Model file for the job. Use its own axes, mm. A direction names the side the tool comes from. Give positions to 0.01 mm unless a question says otherwise; leave off trailing zeros. Write each loop counter-clockwise with the first axis right and the second up, starting at its lowest first coordinate (ties: lowest second). Pieces come first, ordered by that corner, then holes.
```python
from build123d import *

# Parameters (mm, degrees)
SKETCH1_W           = 25.4
SKETCH1_H           = 46.164
BOSS_EXTRUDE1_DEPTH = 6.88
SKETCH2_W           = 13.76
SKETCH2_H           = 15
BOSS_EXTRUDE2_DEPTH = 6.88
SKETCH3_R           = 2.55
CUT_EXTRUDE1_DEPTH  = 7.88
CHAMFER1_SIZE       = 2
FILLET1_R           = 2


with BuildPart() as part:
    # Sketch1 → Boss-Extrude1 (new body)
    with BuildSketch(Plane.XY):
        Rectangle(SKETCH1_W, SKETCH1_H)
    extrude(amount=-BOSS_EXTRUDE1_DEPTH)

    # Sketch2 → Boss-Extrude2 (add)
    with BuildSketch(Plane.XY):
        with Locations((-12.7, 0)):
            Rectangle(SKETCH2_W, SKETCH2_H)
    boss_extrude2 = extrude(amount=-BOSS_EXTRUDE2_DEPTH)

    # Mirror2: Boss-Extrude2 across plane
    add(boss_extrude2.mirror(Plane(origin=(0, 0, 0), x_dir=(0, 0, 1), z_dir=(1, 0, 0))))

    # Sketch3 → Cut-Extrude1 (cut, through all)
    with BuildSketch(Plane.XY):
        Circle(SKETCH3_R)
    extrude(amount=-CUT_EXTRUDE1_DEPTH, mode=Mode.SUBTRACT)

    # Chamfer1
    chamfer1_edges = [part.edges().sort_by_distance(p)[0] for p in [
        (-19.58, -7.5, -3.44),
        (-19.58, 7.5, -3.44),
        (19.58, 7.5, -3.44),
        (19.58, -7.5, -3.44),
        (-12.7, 23.082, -3.44),
        (12.7, 23.082, -3.44),
        (12.7, -23.082, -3.44),
        (-12.7, -23.082, -3.44),
    ]]
    chamfer(chamfer1_edges, length=CHAMFER1_SIZE)

    # Fillet1
    fillet1_edges = [part.edges().sort_by_distance(p)[0] for p in [
        (10.7, 23.082, -3.44),
        (-10.7, 23.082, -3.44),
        (-12.7, 21.082, -3.44),
        (-17.58, 7.5, -3.44),
        (-19.58, -5.5, -3.44),
        (-19.58, 5.5, -3.44),
        (-17.58, -7.5, -3.44),
        (-12.7, -21.082, -3.44),
        (10.7, -23.082, -3.44),
        (-10.7, -23.082, -3.44),
        (12.7, -21.082, -3.44),
        (17.58, -7.5, -3.44),
        (19.58, 5.5, -3.44),
        (19.58, -5.5, -3.44),
        (12.7, 21.082, -3.44),
        (17.58, 7.5, -3.44),
    ]]
    fillet(fillet1_edges, radius=FILLET1_R)


solid = part.part
```
1. Slice it at D-D, the plane x = 14.5. Write the cut outline in (y, z), and give its area (3 significant figures).
Calculated:
outline: (-7.5, -6.88) - (7.5, -6.88) - (7.5, 0) - (-7.5, 0) - close
area: 103 mm2
2. Probe probe 1 along Y at (x, z) = (0, -5); probe 2 along X at (y, z) = (-9, -6.25); probe 3 along Y at (x, z) = (14, -1). List the from-to ranges inside material, lowest first.
Calculated:
probe 1: y = -23.08 to -2.55, 2.55 to 23.08
probe 2: x = -12.7 to 12.7
probe 3: y = -7.5 to 7.5
3. Pin check, flat tips, straight feed: P1, Ø2, axis at x = -13.5, z = -3.5, coming from the -Y side; P2, Ø2, axis at x = 14, z = -5, coming from the +Y side. Stop position of each tip, or through.
Calculated:
P1: stops at y = -21.13
P2: stops at y = 7.5
4. Slice it at B-B, the plane x = 0. Write the cut outline in (y, z).
Calculated:
outline: (-23.08, -6.88) - (-2.55, -6.88) - (-2.55, 0) - (-23.08, 0) - close; (2.55, -6.88) - (23.08, -6.88) - (23.08, 0) - (2.55, 0) - close
5. Slice it at C-C, the plane y = -14.5. Write the cut outline in (x, z).
Calculated:
outline: (-12.7, -6.88) - (12.7, -6.88) - (12.7, 0) - (-12.7, 0) - close
6. Which spindle directions (+Z, -Z, +X, -X, +Y, -Y) get a long thin tool onto all of the face, cutting with end or side? Do faces 1 (the flat face through (15, -7.5, -3)), 2 (the flat face through (-15, -7.5, -3)), 3 (the flat face through (-12.7, 14, -3)), 4 (the flat face through (15, 7.5, -3)). Say none if no direction does.
Calculated:
face 1: +Z, -Z, +X, -Y
face 2: +Z, -Z, -X, -Y
face 3: +Z, -Z, -X, +Y
face 4: +Z, -Z, +X, +Y
7. Slice it at A-A, the plane y = 0. Write the cut outline in (x, z).
Calculated:
outline: (-19.58, -6.88) - (-2.55, -6.88) - (-2.55, 0) - (-19.58, 0) - close; (2.55, -6.88) - (19.58, -6.88) - (19.58, 0) - (2.55, 0) - close
